Autodesk Fusion 360 part; units mm, degrees
sketch "Sketch1" plane through (0, 0, 0) normal (0, 0, 1) x (1, 0, 0)
  line L0 (18.6978, -81.3757) -> (27.6301, -17.0635)
  line L1 (12.7727, 0) -> (-12.7727, 0)
  line L2 (-27.6301, -17.0635) -> (-18.6978, -81.3757)
  line L3 (-8.7929, -90) -> (8.7929, -90)
  arc A0 (-12.7727, 0) -> (-27.6301, -17.0635) centre (-12.7727, -15) ccw
  arc A1 (27.6301, -17.0635) -> (12.7727, 0) centre (12.7727, -15) ccw
  arc A2 (-18.6978, -81.3757) -> (-8.7929, -90) centre (-8.7929, -80) ccw
  arc A3 (8.7929, -90) -> (18.6978, -81.3757) centre (8.7929, -80) ccw
  line L4 (10.5, -78) -> (-10.5, -78)
  line L5 (-12.5, -80) -> (-12.5, -82)
  line L6 (-10.5, -84) -> (10.5, -84)
  line L7 (12.5, -82) -> (12.5, -80)
  arc A4 (-10.5, -78) -> (-12.5, -80) centre (-10.5, -80) ccw
  arc A5 (12.5, -80) -> (10.5, -78) centre (10.5, -80) ccw
  arc A6 (-12.5, -82) -> (-10.5, -84) centre (-10.5, -82) ccw
  arc A7 (10.5, -84) -> (12.5, -82) centre (10.5, -82) ccw
  line L8 (14.3727, -39.8254) -> (16.9352, -21.3757)
  line L9 (7.0302, -10) -> (-7.0302, -10)
  line L10 (-16.9352, -21.3757) -> (-14.3727, -39.8254)
  line L11 (-8.4297, -45) -> (8.4297, -45)
  arc A8 (-7.0302, -10) -> (-16.9352, -21.3757) centre (-7.0302, -20) ccw
  arc A9 (16.9352, -21.3757) -> (7.0302, -10) centre (7.0302, -20) ccw
  arc A10 (8.4297, -45) -> (14.3727, -39.8254) centre (8.4297, -39) ccw
  arc A11 (-14.3727, -39.8254) -> (-8.4297, -45) centre (-8.4297, -39) ccw
  point P0 (17.5, -90)
  point P1 (30, 0)
  point P2 (-30, 0)
  point P3 (-17.5, -90)
  point P4 (12.5, -78)
  point P5 (-12.5, -78)
  point P6 (12.5, -84)
  dimension "d3" = 90
  dimension "d4" = 60
  dimension "d5" = 35
  dimension "d9" = 12.5
  dimension "d10" = 15
  dimension "d11" = 15
  dimension "d12" = 10
  dimension "d13" = 10
  dimension "d14" = 25
  dimension "d15" = 6
  dimension "d16" = 6
  dimension "d17" = 2
  dimension "d18" = 2
  dimension "d19" = 2
  dimension "d20" = 2
  dimension "d21" = 12.5
  dimension "d22" = 10
  dimension "d23" = 10
  dimension "d24" = 6
  dimension "d25" = 6
  dimension "d26" = 10
  dimension "d27" = 10
  dimension "d28" = 10
  dimension "d29" = 35
extrude "Extrude1" add sketch "Sketch1" along normal blind 15
extrude "Extrude2" cut 1 faces at (2.8099, -67, 15) along direction (0, 0, -1) blind 3
extrude "Extrude3" cut 1 faces at (2.8099, -67, 12) along direction (0, 0, -1) blind 2
sketch "Sketch2" plane through (0, -45, 0) normal (0, 1, 0) x (-1, 0, 0)
  line L0 (8.4297, 10) -> (-8.4297, 10)
  line L1 (-8.4297, 10) -> (-8.4297, 0)
  line L2 (-8.4297, 0) -> (8.4297, 0)
  line L3 (8.4297, 0) -> (8.4297, 10)
  line L4 (12.5, 5.75) -> (-12.5, 5.75)
  line L5 (-12.5, 5.75) -> (-12.5, 4.25)
  line L6 (-12.5, 4.25) -> (12.5, 4.25)
  line L7 (12.5, 4.25) -> (12.5, 5.75)
  point P0 (-12.7727, 10)
  dimension "d36" = 25
  dimension "d37" = 1.5
  dimension "d38" = 12.5
  dimension "d39" = 4.25
extrude "Extrude4" cut sketch "Sketch2" along normal blind 3 and the other way blind 15 contours L3 L4 L6 L7 | L1 L3 L4 L6 | L1 L4 L5 L6
sketch "Sketch3" plane through (0, 0, 10) normal (0, 0, 1) x (-1, 0, 0)
  arc A0 (-10.5, 84) -> (-12.5, 82) centre (-10.5, 82) ccw
  line L0 (-10.5, 84) -> (10.5, 84)
  arc A1 (12.5, 82) -> (10.5, 84) centre (10.5, 82) ccw
  line L1 (12.5, 82) -> (12.5, 80)
  arc A2 (10.5, 78) -> (12.5, 80) centre (10.5, 80) ccw
  line L2 (10.5, 78) -> (-10.5, 78)
  arc A3 (-12.5, 80) -> (-10.5, 78) centre (-10.5, 80) ccw
  line L3 (-12.5, 80) -> (-12.5, 82)
  arc A4 (14.3727, 39.8254) -> (8.4297, 45) centre (8.4297, 39) ccw
  line L4 (14.3727, 39.8254) -> (16.9352, 21.3757)
  arc A5 (7.0302, 10) -> (16.9352, 21.3757) centre (7.0302, 20) ccw
  line L5 (7.0302, 10) -> (-7.0302, 10)
  arc A6 (-16.9352, 21.3757) -> (-7.0302, 10) centre (-7.0302, 20) ccw
  line L6 (-16.9352, 21.3757) -> (-14.3727, 39.8254)
  arc A7 (-8.4297, 45) -> (-14.3727, 39.8254) centre (-8.4297, 39) ccw
  line L7 (-8.4297, 45) -> (8.4297, 45)
  arc A8 (-8.7929, 90) -> (-18.6978, 81.3757) centre (-8.7929, 80) ccw
  line L8 (-18.6978, 81.3757) -> (-27.6301, 17.0635)
  arc A9 (-27.6301, 17.0635) -> (-12.7727, 0) centre (-12.7727, 15) ccw
  line L9 (-12.7727, 0) -> (12.7727, 0)
  arc A10 (12.7727, 0) -> (27.6301, 17.0635) centre (12.7727, 15) ccw
  line L10 (27.6301, 17.0635) -> (18.6978, 81.3757)
  arc A11 (18.6978, 81.3757) -> (8.7929, 90) centre (8.7929, 80) ccw
  line L11 (8.7929, 90) -> (-8.7929, 90)
equation "D_krona = 25 mm"
equation "d3 = haed"
equation "d4 = max_b"
equation "d5 = min_b"
equation "max_b = 60 mm"
equation "min_b = 35 mm"
equation "haed = 90 mm"
equation "d9 = ( max_b - min_b ) / 2"
equation "d14 = D_krona"
equation "d21 = D_krona / 2"
equation "d36 = D_krona"
equation "d37 = Linear Dimension-3"
equation "d38 = D_krona / 2"
equation "d39 = Linear Dimension-5"
equation "d42 = D_krona - 10 mm"
Work out the finished part from the listing and answer in its coordinate system (mm). A direction names the side the tool comes from. Give positions to 0.01 mm unless a question says otherwise; leave off trailing zeros. Write each loop counter-clockwise with the first axis right and the second up, starting at its lowest first coordinate (ties: lowest second). Pieces come first, ordered by that corner, then holes. Notation, with made-up numbers: (38, -4.5) - (60, -4.5) arc R19 cw to (60, 17.5) - close; hole circle Ø3 at (52.5, -31). An arc over 180 degrees is marked (long way). Use one line per item in the form item = value.
1. A cutting plane is placed at B-B (z = 9). Write down the section's boundary in (x, y), and give its area (3 significant figures).
Filled in:
outline = (-27.63, -17.06) - (-18.7, -81.38) arc R10 ccw to (-8.79, -90) - (8.79, -90) arc R10 ccw to (18.7, -81.38) - (27.63, -17.06) arc R15 ccw to (12.77, 0) - (-12.77, 0) arc R15 ccw to start; hole (-16.94, -21.38) - (-14.37, -39.83) arc R6 ccw to (-8.43, -45) - (8.43, -45) arc R6 ccw to (14.37, -39.83) - (16.94, -21.38) arc R10 ccw to (7.03, -10) - (-7.03, -10) arc R10 ccw to start; hole (-12.5, -82) arc R2 ccw to (-10.5, -84) - (10.5, -84) arc R2 ccw to (12.5, -82) - (12.5, -80) arc R2 ccw to (10.5, -78) - (-10.5, -78) arc R2 ccw to (-12.5, -80) - close
area = 2,910 mm^2
2. A cutting plane is placed at A-A (y = -37). Write down the section's boundary in (x, z).
Filled in:
outline = (-24.86, 0) - (-14.77, 0) - (-14.77, 10) - (-24.86, 10) - close; (14.77, 0) - (24.86, 0) - (24.86, 10) - (14.77, 10) - close
3. A cutting plane is placed at D-D (y = -46.5). Write down the section's boundary in (x, z).
Filled in:
outline = (-23.54, 0) - (23.54, 0) - (23.54, 10) - (-23.54, 10) - close; hole (-12.5, 4.25) - (12.5, 4.25) - (12.5, 5.75) - (-12.5, 5.75) - close
4. Consider L1, parallel to Y at x = 4, z = 6.25; L2, parallel to Y at x = -12, z = 2.5; L3, parallel to X at y = -79, z = 9. Determine where each line is inside the solid, lowest interval first.
Filled in:
L1 = -90 to -84, -78 to -45, -10 to 0
L2 = -89.47 to -83.32, -78.68 to -43.82, -11.32 to 0
L3 = -19.03 to -12.23, 12.23 to 19.03
5. Each of these flat-tipped pins is pushed along its axis until it touches: pin 1 Ø3 at (y, z) = (-49, 7) entering from -X; pin 2 Ø1 at (y, z) = (-81, 7.5) entering from +X; pin 3 Ø5 at (y, z) = (-76, 6.5) entering from -X. Where does it stop, or does it pass through?
Filled in:
pin_1 = -23.4
pin_2 = 18.82
pin_3 = -19.79
6. Determine the mould class of faces 3 (the face through (0, -52, 4.25)), 4 (the face through (0, -90, 5)), 5 (the face through (0, -54, 0)) for opening direction Z: released by +Z, released by -Z, zero draft, split by the parting line, or undercut.
Filled in:
face_3 = undercut
face_4 = zero draft
face_5 = released by -Z
7. A cutting plane is placed at C-C (y = -57). Write down the section's boundary in (x, z), and give its area (3 significant figures).
Filled in:
outline = (-22.08, 0) - (22.08, 0) - (22.08, 10) - (-22.08, 10) - close; hole (-12.5, 4.25) - (12.5, 4.25) - (12.5, 5.75) - (-12.5, 5.75) - close
area = 404 mm^2
8. For faces 1 (the face through (-11.9, -83.43, 4.93)), 2 (the face through (23.1, -49.67, 4.93)), determine the directions among +Z, -Z, +X, -X, +Y, -Y from which every point of the face is accessible in a straight line to the end or side of a thin tool.
Filled in:
face_1 = +Z, -Z
face_2 = +Z, -Z, +X, -Y
